from build123d import *

# Parameters (mm, degrees)
SALIENTE_EXTRUIR1_DEPTH    = 10
CROQUIS2_W                 = 5
CROQUIS2_H                 = 45
CORTAR_EXTRUIR1_DEPTH      = 12.5
CROQUIS4_W                 = 73.322426794
CROQUIS4_H                 = 5
SALIENTE_EXTRUIR2_DEPTH    = 30
CROQUIS5_W                 = 2.5
CROQUIS5_H                 = 5
SALIENTE_EXTRUIR3_DEPTH    = 50
CROQUIS6_W                 = 55.637494131
CROQUIS6_H                 = 64.414873678
CORTAR_EXTRUIR2_DEPTH      = 55
CROQUIS7_R                 = 1.5
CORTAR_EXTRUIR3_DEPTH      = 5
CROQUIS8_W                 = 39.981329184
CROQUIS8_H                 = 5
CORTAR_EXTRUIR4_DEPTH      = 10
CROQUIS9_W                 = 10
CROQUIS9_H                 = 7.5
SALIENTE_EXTRUIR4_DEPTH    = 21
CROQUIS11_R                = 2
CORTAR_EXTRUIR5_DEPTH      = 21
SALIENTE_EXTRUIR5_START    = -40
CROQUIS12_W                = 21.008716652
CROQUIS12_H                = 5
SALIENTE_EXTRUIR5_DEPTH    = 40
CORTAR_EXTRUIR6_DEPTH      = 62.200166864
CROQUIS15_W                = 5
CROQUIS15_H                = 10
SALIENTE_EXTRUIR6_DEPTH    = 31.1
SALIENTE_EXTRUIR7_DEPTH    = 10
SALIENTE_EXTRUIR8_DEPTH    = 5
CORTAR_EXTRUIR7_START      = -13
CROQUIS21_R                = 1.5
CORTAR_EXTRUIR7_DEPTH      = 13
CORTAR_EXTRUIR10_START     = -52.1
CORTAR_EXTRUIR10_OUTLINE_W = 10
CORTAR_EXTRUIR10_OUTLINE_H = 7.5
CORTAR_EXTRUIR10_DEPTH     = 52.1
SALIENTE_EXTRUIR9_DEPTH    = 10
CROQUIS24_R                = 2
CORTAR_EXTRUIR11_DEPTH     = 10


# Read off the part's stored shape, not the designer's step: Cortar-Extruir10
with BuildPart() as part:
    # Croquis1 → Saliente-Extruir1 (new body)
    with BuildSketch(Plane.XY):
        with BuildLine():
            Line((-35, 10), (-35, 0))
            Line((-35, 0), (-30, 0))
            Line((-30, 0), (-30, 10))
            Line((-30, 10), (-20, 10))
            Line((-20, 10), (-20, 35.723707224))
            ThreePointArc((-20, 35.723707224), (0, 55.723707224), (20, 35.723707224))
            Line((20, 35.723707224), (20, 10))
            Line((20, 10), (30, 10))
            Line((30, 10), (30, 0))
            Line((30, 0), (35, 0))
            Line((35, 0), (35, 10))
            Line((35, 10), (39, 10))
            Line((39, 10), (39, 20))
            Line((39, 20), (14.443351433, 84.048407017))
            Line((14.443351433, 84.048407017), (13.447706691, 86.645237749))
            ThreePointArc((13.447706691, 86.645237749), (0, 95), (-13.447706691, 86.645237749))
            Line((-13.447706691, 86.645237749), (-14.443351433, 84.048407017))
            Line((-14.443351433, 84.048407017), (-39, 20))
            Line((-39, 20), (-39, 10))
            Line((-39, 10), (-35, 10))
        make_face()
        with BuildLine():
            ThreePointArc((1.5, 60), (0, 58.5), (-1.5, 60))
            Line((-1.5, 60), (-1.5, 80))
            ThreePointArc((-1.5, 80), (0, 81.5), (1.5, 80))
            Line((1.5, 80), (1.5, 60))
        make_face(mode=Mode.SUBTRACT)
    extrude(amount=SALIENTE_EXTRUIR1_DEPTH)

    # Croquis2 → Cortar-Extruir1 (cut, symmetric)
    with BuildSketch(Plane(origin=(0, 0, 0), x_dir=(0, 0, -1), z_dir=(1, 0, 0))):
        with Locations((-5, 72.5)):
            Rectangle(CROQUIS2_W, CROQUIS2_H)
    extrude(amount=CORTAR_EXTRUIR1_DEPTH, both=True, mode=Mode.SUBTRACT)

    # Croquis4 → Saliente-Extruir2 (add)
    with BuildSketch(Plane(origin=(0, 0, 0), x_dir=(-1, 0, 0), z_dir=(0, 0, -1))):
        with Locations((0, 28.6)):
            Rectangle(CROQUIS4_W, CROQUIS4_H)
    extrude(amount=SALIENTE_EXTRUIR2_DEPTH)

    # Croquis5 → Saliente-Extruir3 (add)
    with BuildSketch(Plane(origin=(-20, 0, 0), x_dir=(0, 0, -1), z_dir=(1, 0, 0))):
        with Locations((-8.75, 28.6)):
            Rectangle(CROQUIS5_W, CROQUIS5_H)
    extrude(amount=SALIENTE_EXTRUIR3_DEPTH)

    # Croquis6 → Cortar-Extruir2 (cut, symmetric)
    with BuildSketch(Plane(origin=(-20, 0, 0), x_dir=(0, 0, -1), z_dir=(1, 0, 0))):
        with Locations((17.818747066, 63.307436839)):
            Rectangle(CROQUIS6_W, CROQUIS6_H)
    extrude(amount=CORTAR_EXTRUIR2_DEPTH, both=True, mode=Mode.SUBTRACT)

    # Croquis7 → Cortar-Extruir3 (cut)
    with BuildSketch(Plane.XY.offset(10)):
        with Locations((0, 28.6)):
            Circle(CROQUIS7_R)
    extrude(amount=-CORTAR_EXTRUIR3_DEPTH, mode=Mode.SUBTRACT)

    # Croquis8 → Cortar-Extruir4 (cut)
    with BuildSketch(Plane(origin=(0, 31.1, 0), x_dir=(1, 0, 0), z_dir=(0, 1, 0))):
        with Locations((-0.009335408, 2.5)):
            Rectangle(CROQUIS8_W, CROQUIS8_H)
    extrude(amount=-CORTAR_EXTRUIR4_DEPTH, mode=Mode.SUBTRACT)

    # Croquis9 → Saliente-Extruir4 (add)
    with BuildSketch(Plane(origin=(0, 31.1, 0), x_dir=(1, 0, 0), z_dir=(0, 1, 0))):
        with Locations((15.061213397, 24.25)):
            Rectangle(CROQUIS9_W, CROQUIS9_H)
        with Locations((-35.940317185, 24.25)):
            Rectangle(CROQUIS9_W, CROQUIS9_H)
    extrude(amount=SALIENTE_EXTRUIR4_DEPTH)

    # Croquis11 → Cortar-Extruir5 (cut)
    with BuildSketch(Plane.XY.offset(-20.5)):
        with Locations((13.560448106, 46.6)):
            Circle(CROQUIS11_R)
        with Locations((13.560448106, 35.6)):
            Circle(CROQUIS11_R)
        with Locations((-34.439551894, 46.6)):
            Circle(CROQUIS11_R)
        with Locations((-34.439551894, 35.6)):
            Circle(CROQUIS11_R)
    extrude(amount=-CORTAR_EXTRUIR5_DEPTH, mode=Mode.SUBTRACT)

    # Croquis12 → Saliente-Extruir5 (add)
    with BuildSketch(Plane(origin=(0, 0, -30), x_dir=(-1, 0, 0), z_dir=(0, 0, -1)).offset(SALIENTE_EXTRUIR5_START)):
        with Locations((32.834428277, 28.6)):
            Rectangle(CROQUIS12_W, CROQUIS12_H)
    extrude(amount=SALIENTE_EXTRUIR5_DEPTH)

    # Croquis13 → Cortar-Extruir6 (cut, through all)
    with BuildSketch(Plane(origin=(0, 31.1, 0), x_dir=(1, 0, 0), z_dir=(0, 1, 0))):
        Polygon((34.744175198, 0), (36.661213397, 0), (36.661213397, 30), (21.661213397, 30), align=None)
    extrude(amount=-CORTAR_EXTRUIR6_DEPTH, mode=Mode.SUBTRACT)

    # Croquis15 → Saliente-Extruir6 (add)
    with BuildSketch(Plane(origin=(0, 31.1, 0), x_dir=(1, 0, 0), z_dir=(0, 1, 0))):
        with Locations((0, 25)):
            Rectangle(CROQUIS15_W, CROQUIS15_H)
    extrude(amount=-SALIENTE_EXTRUIR6_DEPTH)

    # Croquis18 → Saliente-Extruir7 (add)
    with BuildSketch(Plane.XY.offset(10)):
        Polygon((-39, 10), (-43.338786603, 26.1), (-36.661213397, 26.1), align=None)
    extrude(amount=-SALIENTE_EXTRUIR7_DEPTH)


with BuildPart() as body_2:
    # Croquis20 → Saliente-Extruir8 (new body)
    with BuildSketch(Plane(origin=(0, 31.1, 0), x_dir=(1, 0, 0), z_dir=(0, 1, 0))):
        Polygon((-1.624735856, -15), (1.624735856, -15), (34.744175198, -10), (-43.338786603, -10), align=None)
    extrude(amount=-SALIENTE_EXTRUIR8_DEPTH)

    # Croquis21 → Cortar-Extruir7 (cut)
    with BuildSketch(Plane(origin=(0, 0, 7.5), x_dir=(-1, 0, 0), z_dir=(0, 0, -1)).offset(CORTAR_EXTRUIR7_START)):
        with Locations(Location((0, 28.6, 0), (0, 0, 180))):
            Circle(CROQUIS21_R)
    extrude(amount=CORTAR_EXTRUIR7_DEPTH, mode=Mode.SUBTRACT)


with BuildPart() as cortar_extruir10_tool:
    # Cortar-Extruir10 outline → Cortar-Extruir10 (new body)
    with BuildSketch(Plane(origin=(0, 52.1, 0), x_dir=(1, 0, 0), z_dir=(0, 1, 0)).offset(CORTAR_EXTRUIR10_START)):
        Polygon((1.624735856, -15), (34.744175198, -10), (39, -10), (39, 0), (34.744175198, 0), (21.661213397, 30), (-43.338786603, 30), (-43.338786603, -10), (-1.624735856, -15), align=None)
        Polygon((20, -7.5), (-20, -7.5), (-20, 5), (19.981329184, 5), (19.981329184, 0), (20, 0), align=None, mode=Mode.SUBTRACT)
        with Locations((15.061213397, 24.25)):
            Rectangle(CORTAR_EXTRUIR10_OUTLINE_W, CORTAR_EXTRUIR10_OUTLINE_H, mode=Mode.SUBTRACT)
    extrude(amount=CORTAR_EXTRUIR10_DEPTH)


with BuildPart() as part_1:
    add(part.part)

    # Cortar-Extruir10: cut by cortar_extruir10_tool
    add(cortar_extruir10_tool.part, mode=Mode.SUBTRACT)

    # Croquis23 → Saliente-Extruir9 (add)
    with BuildSketch(Plane.ZY.offset(-10.061213397)):
        Polygon((-28, 31.1), (-35.5, 31.1), (-28, 52.1), align=None)
    extrude(amount=-SALIENTE_EXTRUIR9_DEPTH)

    # Croquis24 → Cortar-Extruir11 (cut)
    with BuildSketch(Plane.XY.offset(-28)):
        with Locations((13.560448106, 46.6)):
            Circle(CROQUIS24_R)
        with Locations((13.560448106, 35.6)):
            Circle(CROQUIS24_R)
    extrude(amount=-CORTAR_EXTRUIR11_DEPTH, mode=Mode.SUBTRACT)


with BuildPart() as body_2_1:
    add(body_2.part)

    # Cortar-Extruir10: cut by cortar_extruir10_tool
    add(cortar_extruir10_tool.part, mode=Mode.SUBTRACT)


solid = part_1.part
The listing builds one solid part. Answer for the finished solid, in the listing's coordinates (mm). A direction names the side the tool comes from. Coordinates: 2 decimals unless noted, no trailing zeros. Order: outer loops, then holes, each group sorted by start corner. A loop starts at its lowest first (then second) coordinate and runs counter-clockwise, first axis right, second up.
Q1. A cutting plane is placed at C-C, the plane x = 16.5. Write down the section's boundary in (y, z).
Q2. A cutting plane is placed at B-B, the plane z = -28.5. Write down the section's boundary in (x, y), and give its area (3 significant figures).
Q3. A cutting plane is placed at D-D, the plane y = 35.6. Write down the section's boundary in (x, z).
Q4. A cutting plane is placed at A-A, the plane y = 46.6. Write down the section's boundary in (x, z).
Q5. Given P1, Ø3, axis at x = 13.56, y = 35.6, coming from the -Z side; P2, Ø4, axis at x = 17, z = -31.5, coming from the -Y side; P3, Ø6, axis at x = 18, y = 34, coming from the -Z side, each flat-ended and moving along its own axis, determine where each tip first touches the part or whether it passes through.
Q6. For a pull along X with two mould halves and no side action, classify faces 3 (the face through (10.061, 39, -26)), 4 (the face through (13.127, 33.648, -27.526)), 5 (the face through (15, 29, -28)) as pulls with the +X half, pulls with the -X half, needs draft (parallel to the pull), parting line crosses it, or undercut.
Q7. Consider line 1 (Y direction, x = 13.5, z = -26.5); line 2 (X direction, y = 35.6, z = -30); line 3 (Y direction, x = 12.25, z = -23.75). Determine where each line is inside the solid, lowest interval first.
Q8. Which of the six approach directions +Z, -Z, +X, -X, +Y, -Y give full straight-line access (tool end or side, diameter ignored) to faces 1 (the face through (15, 31.1, -32)), 2 (the face through (20.061, 39, -26))?
Answers follow:
1. outline: (26.1, -28) - (31.1, -28) - (31.1, -35.5) - (52.1, -28) - (52.1, -20.5) - (26.1, -20.5) - close
2. outline: (10.06, 31.1) - (20.06, 31.1) - (20.06, 50.7) - (10.06, 50.7) - close; hole circle Ø4 at (13.56, 35.6); hole circle Ø4 at (13.56, 46.6)
2. area: 171 mm2
3. outline: (10.06, -33.89) - (11.56, -33.89) - (11.56, -20.5) - (10.06, -20.5) - close; (15.56, -33.89) - (20.06, -33.89) - (20.06, -20.5) - (15.56, -20.5) - close
4. outline: (10.06, -29.96) - (11.56, -29.96) - (11.56, -20.5) - (10.06, -20.5) - close; (15.56, -29.96) - (20.06, -29.96) - (20.06, -20.5) - (15.56, -20.5) - close
5. P1: passes through
5. P2: stops at y = 31.1
5. P3: stops at z = -35.5
6. face 3: pulls with the -X half
6. face 4: undercut
6. face 5: needs draft
7. line 1: y = 26.1 to 33.6, 37.6 to 44.6, 48.6 to 52.1
7. line 2: x = 10.06 to 11.56, 15.56 to 20.06
7. line 3: y = 26.1 to 34.09, 37.11 to 45.09, 48.11 to 52.1
8. face 1: -Z, +X, -X, -Y
8. face 2: +Z, -Z, +X, +Y, -Y
